Verification items for the finished model (mm, model axes). Face numbers are marked on the shaded views. Coordinates: 2 decimals unless noted, no trailing zeros. Loops run counter-clockwise (first coordinate to the right, second up) from the corner with the lowest first, then second, coordinate; pieces in that order, holes last. Notation, with made-up numbers: (19.25, -25) - (43.25, -25) arc R18 ccw to (43.25, 5) - close; hole circle Ø7 at (41.5, 2.5). An arc over 180 degrees is marked (long way). Answer as CSV lines item,"result". Start each with the question number.
1. Cross-section at A-A (z = 21). Enter the section's corners in (x, y), plus the area to 3 significant figures.
2. Material ranges on line 1 (X direction, y = -17, z = 17.5); line 2 (X direction, y = -15, z = 4); line 3 (Z direction, x = -13, y = 15), recorded low to high. Write a range as [from, to].
3. Cross-section at D-D (z = 3). Enter the section's corners in (x, y).
4. Gauge pin test, flat end, axial feed: P1, Ø2, axis at x = 6, y = 13.5, coming from the -Z side. Record the tip position at first contact, or that the pin passes through.
5. Release check for a two-part mould opening along X. For the marked faces 1, 2 and 3 record: pulls with the +X half, pulls with the -X half, needs draft (parallel to the pull), parting line crosses it, or undercut.
6. Cross-section at C-C (x = 0). Enter the section's corners in (y, z), plus the area to 3 significant figures.
7. Cross-section at B-B (y = 13.5). Enter the section's corners in (x, z).
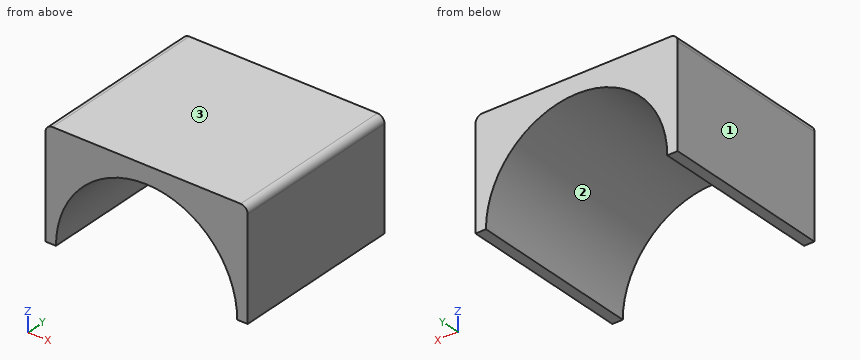
```python
from build123d import *

# Parameters (mm, degrees)
CYLINDER_R     = 26
CYLINDER_DEPTH = 50
BOX_W          = 58
BOX_H          = 50
BOX_DEPTH      = 31
FILLET_R       = 2


with BuildPart() as cylinder:
    # Cylinder → Cylinder (new body)
    with BuildSketch(Plane.XZ.offset(-25)):
        Circle(CYLINDER_R)
    extrude(amount=CYLINDER_DEPTH)


with BuildPart() as obj1:
    # Box → Box (new body)
    with BuildSketch(Plane(origin=(-29, -25, 0), x_dir=(1, 0, 0), z_dir=(0, 0, 1))):
        with Locations((29, 25)):
            Rectangle(BOX_W, BOX_H)
    extrude(amount=BOX_DEPTH)

    # Fillet
    fillet_edges = [obj1.edges().sort_by_distance(p)[0] for p in [
        (-29, 0, 31),
        (29, 0, 31),
    ]]
    fillet(fillet_edges, radius=FILLET_R)

    # Cut: cut Cylinder
    add(cylinder.part, mode=Mode.SUBTRACT)


solid = obj1.part
```
Values follow:
1,outline,"(-29, -25) - (-15.33, -25) - (-15.33, 25) - (-29, 25) - close; (15.33, -25) - (29, -25) - (29, 25) - (15.33, 25) - close"
1,area,"1,370 mm²"
2,line 1,"x = [-29, -19.23], [19.23, 29]"
2,line 2,"x = [-29, -25.69], [25.69, 29]"
2,line 3,"z = [22.52, 31]"
3,outline,"(-29, -25) - (-25.83, -25) - (-25.83, 25) - (-29, 25) - close; (25.83, -25) - (29, -25) - (29, 25) - (25.83, 25) - close"
4,P1,"stops at z = 25.04"
5,face 1,"pulls with the -X half"
5,face 2,"undercut"
5,face 3,"needs draft"
6,outline,"(-25, 26) - (25, 26) - (25, 31) - (-25, 31) - close"
6,area,"250 mm²"
7,outline,"(-29, 0) - (-26, 0) arc R26 cw to (26, 0) - (29, 0) - (29, 29) arc R2 ccw to (27, 31) - (-27, 31) arc R2 ccw to (-29, 29) - close"
